Here's how the part is built. I have some questions about the finished solid (model axes, mm). Face numbers are marked on the shaded views. A direction names the side the tool comes from. Round coordinates to 2 decimals unless told otherwise and drop trailing zeros. Write each loop counter-clockwise with the first axis right and the second up, starting at its lowest first coordinate (ties: lowest second). Pieces come first, ordered by that corner, then holes. Notation, with made-up numbers: (-28, 65.25) -> (-23, 65.25) arc R24 ccw to (-23, 98.25) -> close; hole circle Ø3 at (29.25, -27). An arc over 180 degrees is marked (long way). Put each result on its own line as item: value. Start each with the question number.
1) I want a section at C-C, the plane z = -4. List the corners of the cut face in (x, y) for me, then the cut area to 3 significant figures.
2) I want a section at D-D, the plane y = 4.5. Give the number of separate pieces and of enclosed holes in the cut face, then the cut area to 3 significant figures.
3) If I drill on line 1 along X through (y, z) = (12, -7.5); line 2 along Z through (x, y) = (38, 0.5); line 3 along X through (y, z) = (7, -4.25), over which ranges is the centre line in solid material (lowest first)? Write a range as [from, to].
4) Will these pins go through, and if not, where does the flat tip stop? P1, Ø8, axis at x = 18.5, z = -6.5, coming from the +Y side; P2, Ø1.5, axis at y = 7, z = 0.5, coming from the -X side; P3, Ø8, axis at x = 20.5, z = -6.5, coming from the -Y side.
5) I want a section at A-A, the plane y = 25. List the corners of the cut face in (x, z) for me.
6) We'd pull the mould along Y, two halves only. Please class the marked faces 1, 2 and 3: released by +Y, released by -Y, zero draft, split by the parting line, or undercut.
7) Which directions (+Z, -Z, +X, -X, +Y, -Y) give clear straight access to the entire face, cutting with the end or side of a thin tool? Please do the marked faces 4, 5 and 6.
8) I want a section at B-B, the plane x = 5. List the corners of the cut face in (y, z) for me.
from build123d import *

# Parameters (mm, degrees)
SKETCH_R        = 2
PAD_DEPTH       = 5
SKETCH001_R     = 13
PAD001_DEPTH    = 9
SKETCH002_R     = 8
POCKET_DEPTH    = 18.001
SKETCH003_W     = 37.242641
SKETCH003_H     = 5
POCKET001_DEPTH = 41.926514
SKETCH004_R     = 11.25
POCKET002_DEPTH = 13
CHAMFER_SIZE    = 3.1


with BuildPart() as part:
    # Sketch → Pad (new body)
    with BuildSketch(Plane.XY):
        with BuildLine():
            Line((1.414214, 0), (49.84062, 0))
            ThreePointArc((49.84062, 0), (51.688379, 1.234633), (51.254834, 3.414214))
            Line((51.254834, 3.414214), (27.041631, 27.627417))
            ThreePointArc((27.041631, 27.627417), (25.627417, 28.213203), (24.213203, 27.627417))
            Line((0, 3.414214), (24.213203, 27.627417))
            ThreePointArc((0, 3.414214), (-0.433546, 1.234633), (1.414214, 0))
        make_face()
        with Locations((4.414214, 3.25)):
            Circle(SKETCH_R, mode=Mode.SUBTRACT)
        with Locations((46.84062, 3.25)):
            Circle(SKETCH_R, mode=Mode.SUBTRACT)
        with Locations((25.627417, 24.463203)):
            Circle(SKETCH_R, mode=Mode.SUBTRACT)
    extrude(amount=PAD_DEPTH)

    # Sketch001 (on Face10 of Pad) → Pad001 (join, symmetric)
    with BuildSketch(Plane(origin=(0, 0, 0), x_dir=(1, 0, 0), z_dir=(0, 0, -1))):
        with Locations((25.627417, -8.963203)):
            Circle(SKETCH001_R)
    extrude(amount=PAD001_DEPTH, both=True)

    # Sketch002 (on Face15 of Pad001) → Pocket (cut, through all)
    with BuildSketch(Plane(origin=(0, 0, -9), x_dir=(1, 0, 0), z_dir=(0, 0, -1))):
        with Locations((25.627417, -8.963203)):
            Circle(SKETCH002_R)
    extrude(amount=-POCKET_DEPTH, mode=Mode.SUBTRACT)

    # Sketch003 (on Face8 of Pocket) → Pocket001 (cut, through all)
    with BuildSketch(Plane(origin=(27.334524, 27.334524, 0), x_dir=(-0.707107, 0.707107, 0), z_dir=(0.707107, 0.707107, 0))):
        with Locations((-15.207106, 7.5)):
            Rectangle(SKETCH003_W, SKETCH003_H)
    extrude(amount=-POCKET001_DEPTH, mode=Mode.SUBTRACT)

    # Sketch004 (on Face15 of Pocket001) → Pocket002 (cut)
    with BuildSketch(Plane.XY.offset(5)):
        with Locations((25.627417, 8.963203)):
            Circle(SKETCH004_R)
    extrude(amount=-POCKET002_DEPTH, mode=Mode.SUBTRACT)

    # Chamfer
    chamfer_edges = [part.edges().sort_by_distance(p)[0] for p in [
        (14.377417, 8.963203, -8),
    ]]
    chamfer(chamfer_edges, length=CHAMFER_SIZE)


solid = part.part
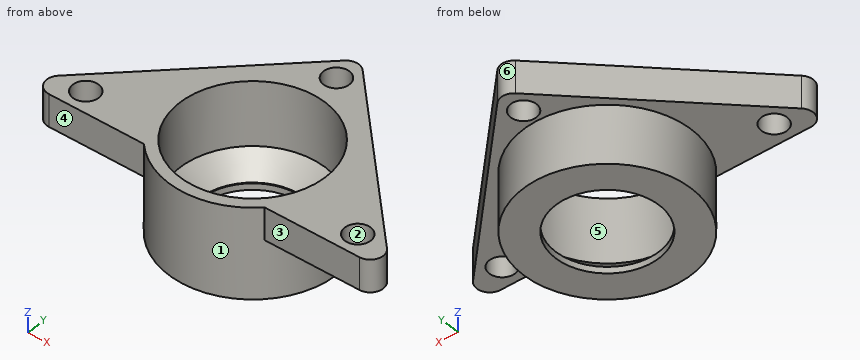
Findings:
1. outline: circle Ø26 at (25.63, 8.96); hole circle Ø22.5 at (25.63, 8.96)
1. area: 133 mm2
2. separate pieces: 4
2. enclosed holes: 0
2. area: 163 mm2
3. line 1: x = [12.99, 17.53], [33.73, 38.27]
3. line 2: z = [0, 5]
3. line 3: x = [12.78, 14.55], [36.7, 38.48]
4. P1: stops at y = 21.58
4. P2: stops at x = 2.84
4. P3: stops at y = -3.99
5. outline: (21.59, 0) -> (23.7, 0) -> (23.7, 5) -> (21.59, 5) -> close; (27.55, 0) -> (29.67, 0) -> (29.67, 5) -> (27.55, 5) -> close
6. face 1: split by the parting line
6. face 2: undercut
6. face 3: released by -Y
7. face 4: +Z, -Z, -X, -Y
7. face 5: +Z
7. face 6: +Z, -Z, +Y
8. outline: (0, 0) -> (1.34, 0) -> (1.34, 5) -> (0, 5) -> close; (5.16, 0) -> (8.41, 0) -> (8.41, 5) -> (5.16, 5) -> close
